For this review, take the finished solid that the model builds, in its own axes (mm). Give positions to 0.01 mm unless a question says otherwise; leave off trailing zeros. Write each loop counter-clockwise with the first axis right and the second up, starting at its lowest first coordinate (ties: lowest second). Pieces come first, ordered by that corner, then holes. Notation, with made-up numbers: (-14, 21) -> (19, 21) arc R28 cw to (19, 56) -> close; hole circle Ø4 at (-21, 18.25). An arc over 180 degrees is marked (long way). Write item = value, one per line.
```python
from build123d import *

# Parameters (mm, degrees)
SKETCH_R              = 3
SKETCH_R_2            = 15.5
PAD_DEPTH             = 6
SKETCH001_R           = 2.5
POCKET_DEPTH          = 10
POLARPATTERN_COUNT    = 4
SKETCH002_R           = 5
POCKET001_DEPTH       = 3
POLARPATTERN001_COUNT = 4
SKETCH003_R           = 6
POCKET002_DEPTH       = 3
SKETCH004_R           = 18
POCKET003_DEPTH       = 3
SKETCH010_R           = 2.5
POCKET007_DEPTH       = 6
SKETCH011_R           = 5
POCKET008_DEPTH       = 3
POLARPATTERN004_COUNT = 4
SKETCH012_R           = 2.5
POCKET009_DEPTH       = 6
SKETCH013_R           = 5
POCKET010_DEPTH       = 3


with BuildPart() as part:
    # Sketch → Pad (new body)
    with BuildSketch(Plane.XY):
        with BuildLine():
            ThreePointArc((19.98, 87.7542), (-90, 0), (19.98, -87.7542))
            Line((19.98, -87.7542), (257.659, -33.63911))
            ThreePointArc((257.659, -33.63911), (284.5, 0), (257.659, 33.63911))
            Line((19.98, 87.7542), (257.659, 33.63911))
        make_face()
        with Locations((250, 0)):
            Circle(SKETCH_R, mode=Mode.SUBTRACT)
        Circle(SKETCH_R_2, mode=Mode.SUBTRACT)
    extrude(amount=PAD_DEPTH)

    # Sketch001 (on Face8 of Pad) → Pocket (cut)
    with BuildSketch(Plane.XY.offset(6)):
        with Locations((42.4248, 42.428014)):
            Circle(SKETCH001_R)
    pocket = extrude(amount=-POCKET_DEPTH, mode=Mode.SUBTRACT)

    # PolarPattern: Pocket ×4 about axis
    polarpattern_axis = Axis((0, 0, 6), (0, 0, 1))
    for i in range(1, POLARPATTERN_COUNT):
        add(pocket.rotate(polarpattern_axis, i * 360 / POLARPATTERN_COUNT), mode=Mode.SUBTRACT)

    # Sketch002 (on Face5 of PolarPattern) → Pocket001 (cut)
    with BuildSketch(Plane.XY.offset(6)):
        with Locations((-42.428014, 42.4248)):
            Circle(SKETCH002_R)
    pocket001 = extrude(amount=-POCKET001_DEPTH, mode=Mode.SUBTRACT)

    # PolarPattern001: Pocket001 ×4 about axis
    polarpattern001_axis = Axis((0, 0, 6), (0, 0, 1))
    for i in range(1, POLARPATTERN001_COUNT):
        add(pocket001.rotate(polarpattern001_axis, i * 360 / POLARPATTERN001_COUNT), mode=Mode.SUBTRACT)

    # Sketch003 (on Face5 of PolarPattern001) → Pocket002 (cut)
    with BuildSketch(Plane.XY.offset(6)):
        with Locations((250, 0)):
            Circle(SKETCH003_R)
    extrude(amount=-POCKET002_DEPTH, mode=Mode.SUBTRACT)

    # Sketch004 (on Face5 of Pocket002) → Pocket003 (cut)
    with BuildSketch(Plane.XY.offset(6)):
        Circle(SKETCH004_R)
    extrude(amount=-POCKET003_DEPTH, mode=Mode.SUBTRACT)

    # Sketch010 (on Face5 of Pocket003) → Pocket007 (cut)
    with BuildSketch(Plane.XY.offset(6)):
        with Locations((53, 28)):
            Circle(SKETCH010_R)
        with Locations((53, -28)):
            Circle(SKETCH010_R)
    pocket007 = extrude(amount=-POCKET007_DEPTH, mode=Mode.SUBTRACT)

    # Sketch011 (on Face5 of Pocket007) → Pocket008 (cut)
    with BuildSketch(Plane.XY.offset(6)):
        with Locations((53, 28)):
            Circle(SKETCH011_R)
        with Locations((53, -28)):
            Circle(SKETCH011_R)
    pocket008 = extrude(amount=-POCKET008_DEPTH, mode=Mode.SUBTRACT)

    # PolarPattern004: Pocket007, Pocket008 ×4 about axis
    polarpattern004_axis = Axis((0, 0, 6), (0, 0, 1))
    for i in range(1, POLARPATTERN004_COUNT):
        add(pocket007.rotate(polarpattern004_axis, i * 360 / POLARPATTERN004_COUNT), mode=Mode.SUBTRACT)
        add(pocket008.rotate(polarpattern004_axis, i * 360 / POLARPATTERN004_COUNT), mode=Mode.SUBTRACT)

    # Sketch012 (on Face5 of PolarPattern004) → Pocket009 (cut)
    with BuildSketch(Plane.XY.offset(6)):
        with Locations((28, -25)):
            Circle(SKETCH012_R)
        with Locations((27.5, 20)):
            Circle(SKETCH012_R)
    pocket009 = extrude(amount=-POCKET009_DEPTH, mode=Mode.SUBTRACT)

    # Sketch013 (on Face5 of Pocket009) → Pocket010 (cut)
    with BuildSketch(Plane.XY.offset(6)):
        with Locations((27.5, 20)):
            Circle(SKETCH013_R)
        with Locations((28, -25)):
            Circle(SKETCH013_R)
    pocket010 = extrude(amount=-POCKET010_DEPTH, mode=Mode.SUBTRACT)

    # Mirrored: Pocket010, Pocket009 across Sketch013 V_Axis
    add(pocket010.mirror(Plane(origin=(0, 0, 6), x_dir=(0, 0, 1), z_dir=(1, 0, 0))), mode=Mode.SUBTRACT)
    add(pocket009.mirror(Plane(origin=(0, 0, 6), x_dir=(0, 0, 1), z_dir=(1, 0, 0))), mode=Mode.SUBTRACT)


solid = part.part
```
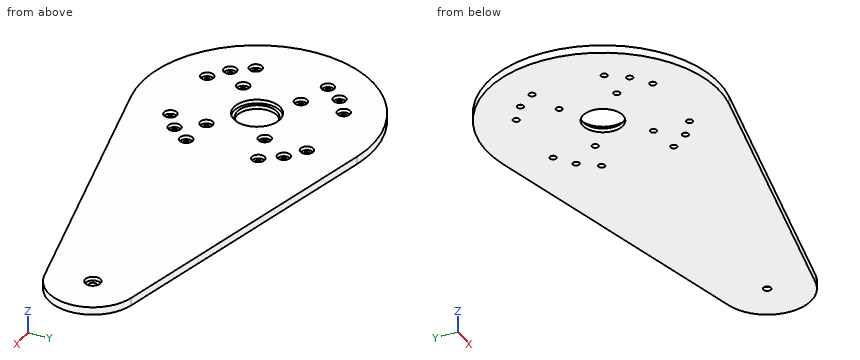
(1) Take a section at C-C (y = 75.5). Write out the cut boundary in (x, z), plus the area to 3 significant figures.
Answers below:
outline = (-48.99, 0) -> (73.8, 0) -> (73.8, 6) -> (-48.99, 6) -> close
area = 737 mm^2
(2) Take a section at B-B (z = 4.9). Count the separate pieces of the cut face and the enclosed holes in it, plus the area to 3 significant figures.
Answers below:
separate_pieces = 1
enclosed_holes = 18
area = 44,100 mm^2
(3) Take a section at A-A (x = -10.5). Write out the cut boundary in (y, z), plus the area to 3 significant figures.
Answers below:
outline = (-89.39, 0) -> (-11.4, 0) -> (-11.4, 3) -> (-14.62, 3) -> (-14.62, 6) -> (-89.39, 6) -> close; (11.4, 0) -> (89.39, 0) -> (89.39, 6) -> (14.62, 6) -> (14.62, 3) -> (11.4, 3) -> close
area = 916 mm^2
(4) To check wall thickness, follow probe 1 along X at (y, z) = (-27, 4.9); probe 2 along Y at (x, z) = (53, 1.5); probe 3 along Z at (x, y) = (-25.5, 56). State the ranges of each line that lie inside material, in increasing order.
Answers below:
probe_1 = -85.85 to -57.9, -48.1 to -32.58, -23.42 to 23.42, 32.58 to 48.1, 57.9 to 271.48
probe_2 = -80.24 to -30.5, -25.5 to 25.5, 30.5 to 80.24
probe_3 = 0 to 3
(5) For pin 1 (4 mm diameter, centred on x = -53, y = 28, fed in from -Z); pin 2 (3 mm diameter, centred on x = -27.5, y = 51.5, fed in from +Z); pin 3 (3 mm diameter, centred on x = 100.5, z = 5, fed in from +Y); pin 4 (1.5 mm diameter, centred on x = 146, z = 3, fed in from +Y), all flat-tipped, find the tip position at first contact; note any pin that passes through.
Answers below:
pin_1 = through
pin_2 = 3
pin_3 = 69.76
pin_4 = 59.23
(6) Take a section at D-D (x = 203.5). Write out the cut boundary in (y, z), plus the area to 3 significant figures.
Answers below:
outline = (-45.97, 0) -> (45.97, 0) -> (45.97, 6) -> (-45.97, 6) -> close
area = 552 mm^2
